```python
from build123d import *

# Parameters (mm, degrees)
EXTRUDE_THIN1_DEPTH = 88.9
CUT_EXTRUDE1_REACH  = 105.954
SKETCH2_R           = 4.7625


with BuildPart() as part:
    # Sketch1 → Extrude-Thin1 (new, symmetric)
    with BuildSketch(Plane(origin=(0, 0, 0), x_dir=(0, 0, -1), z_dir=(1, 0, 0))):
        Polygon((-38.1, 0), (0, 0), (0, 38.1), (-3.175, 38.1), (-3.175, 3.175), (-38.1, 3.175), align=None)
    extrude(amount=EXTRUDE_THIN1_DEPTH, both=True)

    # Sketch2 → Cut-Extrude1 (cut, up to next)
    with BuildSketch(Plane(origin=(0, 0, 0), x_dir=(-1, 0, 0), z_dir=(0, 0, -1)), mode=Mode.PRIVATE) as cut_extrude1_sk1:
        with Locations((-76.2, 25.4)):
            Circle(SKETCH2_R)
    cut_extrude1_tool1 = extrude(cut_extrude1_sk1.sketch, amount=-CUT_EXTRUDE1_REACH, mode=Mode.PRIVATE) & part.part
    # Sketch2 → Cut-Extrude1 (cut, up to next)
    with BuildSketch(Plane(origin=(0, 0, 0), x_dir=(-1, 0, 0), z_dir=(0, 0, -1)), mode=Mode.PRIVATE) as cut_extrude1_sk2:
        with Locations((76.2, 25.4)):
            Circle(SKETCH2_R)
    cut_extrude1_tool2 = extrude(cut_extrude1_sk2.sketch, amount=-CUT_EXTRUDE1_REACH, mode=Mode.PRIVATE) & part.part
    add(cut_extrude1_tool1.solids().sort_by_distance((76.2, 25.4, 0))[0], mode=Mode.SUBTRACT)
    add(cut_extrude1_tool2.solids().sort_by_distance((-76.2, 25.4, 0))[0], mode=Mode.SUBTRACT)


solid = part.part
```
Model file for the job. Use its own axes, mm. A direction names the side the tool comes from. Give positions to 0.01 mm unless a question says otherwise; leave off trailing zeros. Loops run counter-clockwise (first coordinate to the right, second up) from the corner with the lowest first, then second, coordinate; pieces in that order, holes last. Notation, with made-up numbers: M 75,58 L 131,58 A13 ccw 131,76 Z; hole C 71,38 d5. An arc over 180 degrees is marked long. Use one line per item in the form item = value.
Item 1: Slice it at B-B on y = 25.4. List the corners of the cut face in (x, z) (1 decimal), and give its area (3 significant figures).
Filled in:
outline = M -88.9,0 L -81,0 L -81,3.2 L -88.9,3.2 Z; M -71.4,0 L 71.4,0 L 71.4,3.2 L -71.4,3.2 Z; M 81,0 L 88.9,0 L 88.9,3.2 L 81,3.2 Z
area = 504 mm^2
Item 2: Slice it at C-C on z = 28.5. List the corners of the cut face in (x, y) (3 decimals).
Filled in:
outline = M -88.9,0 L 88.9,0 L 88.9,3.175 L -88.9,3.175 Z
Item 3: Flat gauge pins, fed straight in: pin 1 Ø11 at (x, y) = (76.2, 25.4) entering from +Z (3 decimals); pin 2 Ø4 at (x, z) = (-71, 26) entering from +Y (3 decimals). Where does each tip first touch, or does it go through?
Filled in:
pin_1 = 3.175
pin_2 = 3.175
Item 4: Drill centre lines: L1, parallel to Y at x = 76.2, z = 1.8; L2, parallel to X at y = 25, z = 1; L3, parallel to Y at x = -4.5, z = 17 (3 decimals). Where is each one in solid material? Low to high.
Filled in:
L1 = 0 to 20.64, 30.16 to 38.1
L2 = -88.9 to -80.95, -71.45 to 71.45, 80.95 to 88.9
L3 = 0 to 3.175
Item 5: Which spindle directions (+Z, -Z, +X, -X, +Y, -Y) get a long thin tool onto all of the face, cutting with end or side? Do faces 4 (the flat face through (1, 21, 3.175)), 5 (the flat face through (1, 2, 38.1)). Say none if no direction does.
Filled in:
face_4 = +Z, +X, -X, +Y
face_5 = +Z, +X, -X, +Y, -Y
Item 6: Slice it at D-D on x = 7. List the corners of the cut face in (y, z) (3 decimals).
Filled in:
outline = M 0,0 L 38.1,0 L 38.1,3.175 L 3.175,3.175 L 3.175,38.1 L 0,38.1 Z
Item 7: Slice it at A-A on x = 76.2. List the corners of the cut face in (y, z) (1 decimal).
Filled in:
outline = M 0,0 L 20.6,0 L 20.6,3.2 L 3.2,3.2 L 3.2,38.1 L 0,38.1 Z; M 30.2,0 L 38.1,0 L 38.1,3.2 L 30.2,3.2 Z
Item 8: Two-plate mould, pull along X, no slides. Class faces 1 (the cylindrical face through (80.958, 25.609, 1.565)), 2 (the flat face through (1, 0, 19)), 3 (the flat face through (-88.9, 2, 11)): released by +X, released by -X, zero draft, split by the parting line, or undercut.
Filled in:
face_1 = undercut
face_2 = zero draft
face_3 = released by -X
